Autodesk Inventor part; units mm, degrees
ref_plane "YZ Plane" through (0, 0, 0) normal (1, 0, 0) x (0, 1, 0)
ref_plane "XZ Plane" through (0, 0, 0) normal (0, 1, 0) x (-1, 0, 0)
ref_plane "XY Plane" through (0, 0, 0) normal (0, 0, 1) x (1, 0, 0)
sketch "Sketch3" plane through (0, 0, 0) normal (1, 0, 0) x (0, 1, 0)
  line L0 (0, 0) -> (0, -3.6)
  line L1 (0, -3.6) -> (5.5, -3.6)
  line L2 (5.5, -3.6) -> (5.5, -2.55)
  line L3 (5.5, -2.55) -> (10, -2.55)
  line L4 (10, -2.55) -> (10, 0)
  line L5 (10, 0) -> (0, 0)
  dimension "baseRadius" = 3.6
  dimension "d12" = 10
  dimension "d13" = 2.55
  dimension "baseHeight" = 5.5
revolve "Revolution1" add sketch "Sketch3" angle 360 about axis through (0, 10, 0) along (0, -1, 0)
sketch "Sketch4" plane through (0, 10, 0) normal (0, 1, 0) x (1, 0, 0)
  point P0 (0, 0)
hole "Hole2" at (0, 10, 0) direction (0, -1, 0) diameter 2 depth 6 countersink diameter 2.5 countersink angle 70
fillet "Fillet2" radius 1 1 edges at (0, 10, 2.55)
chamfer "Chamfer1" distance 0.6 distance2 1 1 edges at (0, 0, 3.6) measured on face at (0.7957, 0, -0.8982)
properties part number "stylus_nib_base"
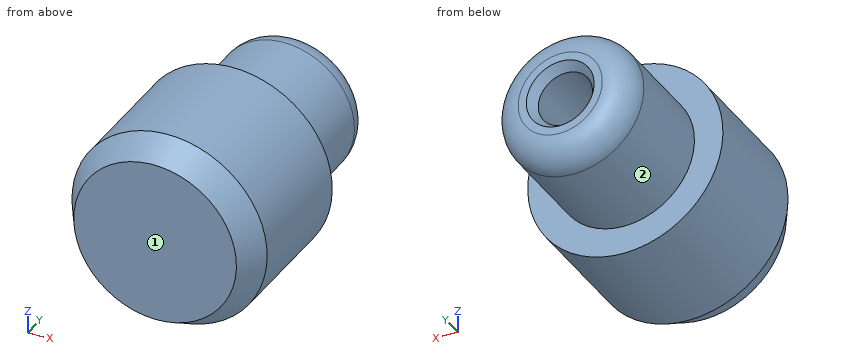
Could you check a few things on this model? Use its own coordinates, in mm. Face numbers are marked on the shaded views. A direction names the side the tool comes from. Give positions to 0.01 mm unless a question says otherwise; leave off trailing zeros. Order: outer loops, then holes, each group sorted by start corner. A loop starts at its lowest first (then second) coordinate and runs counter-clockwise, first axis right, second up.
Q1. Suppose I cut it at B-B, the plane z = 0. Write out the boundary of the cut face in (x, y).
Q2. Suppose I cut it at A-A, the plane y = 4.75. Write out the boundary of the cut face in (x, z).
Q3. For the marked faces 1 and 2, which set-ups out of +Z, -Z, +X, -X, +Y, -Y let a thin tool reach every point of the face, with its end or its side?
Q4. Suppose I cut it at D-D, the plane y = 3. Write out the boundary of the cut face in (x, z), and give its area (3 significant figures).
Q5. Suppose I cut it at C-C, the plane x = 0. Write out the boundary of the cut face in (y, z).
Q6. If I drill on line 1 along X through (y, z) = (7.7, 0); line 2 along Z through (x, y) = (0.75, 7.75); line 3 along X through (y, z) = (5.75, 1.75), over which ranges is the centre line in solid material (lowest first)?
Q7. I'm going to push flat-ended pins straight in: P1, Ø3, axis at y = 9, z = -0.5, coming from the -X side; P2, Ø1.5, axis at y = 2, z = 2.5, coming from the +X side; P3, Ø3, axis at x = 0, z = 0, coming from the +Y side; P4, Ø1.5, axis at y = 9, z = 0.5, coming from the +X side. Where does each tip first touch, or does it pass through?
Solution:
1. outline: (-3.6, 1) - (-3, 0) - (3, 0) - (3.6, 1) - (3.6, 5.5) - (2.55, 5.5) - (2.55, 9) arc R1 ccw to (1.55, 10) - (1.25, 10) - (1, 9.64) - (1, 4) - (-1, 4) - (-1, 9.64) - (-1.25, 10) - (-1.55, 10) arc R1 ccw to (-2.55, 9) - (-2.55, 5.5) - (-3.6, 5.5) - close
2. outline: circle Ø7.2 at (0, 0); hole circle Ø2 at (0, 0)
3. face 1: +Z, -Z, +X, -X, -Y
3. face 2: +Y
4. outline: circle Ø7.2 at (0, 0)
4. area: 40.7 mm2
5. outline: (0, -3) - (1, -3.6) - (5.5, -3.6) - (5.5, -2.55) - (9, -2.55) arc R1 ccw to (10, -1.55) - (10, -1.25) - (9.64, -1) - (4, -1) - (4, 1) - (9.64, 1) - (10, 1.25) - (10, 1.55) arc R1 ccw to (9, 2.55) - (5.5, 2.55) - (5.5, 3.6) - (1, 3.6) - (0, 3) - close
6. line 1: x = -2.55 to -1, 1 to 2.55
6. line 2: z = -2.44 to -0.66, 0.66 to 2.44
6. line 3: x = -1.85 to 1.85
7. P1: stops at x = -2.55
7. P2: stops at x = 3.15
7. P3: stops at y = 10
7. P4: stops at x = 2.55
